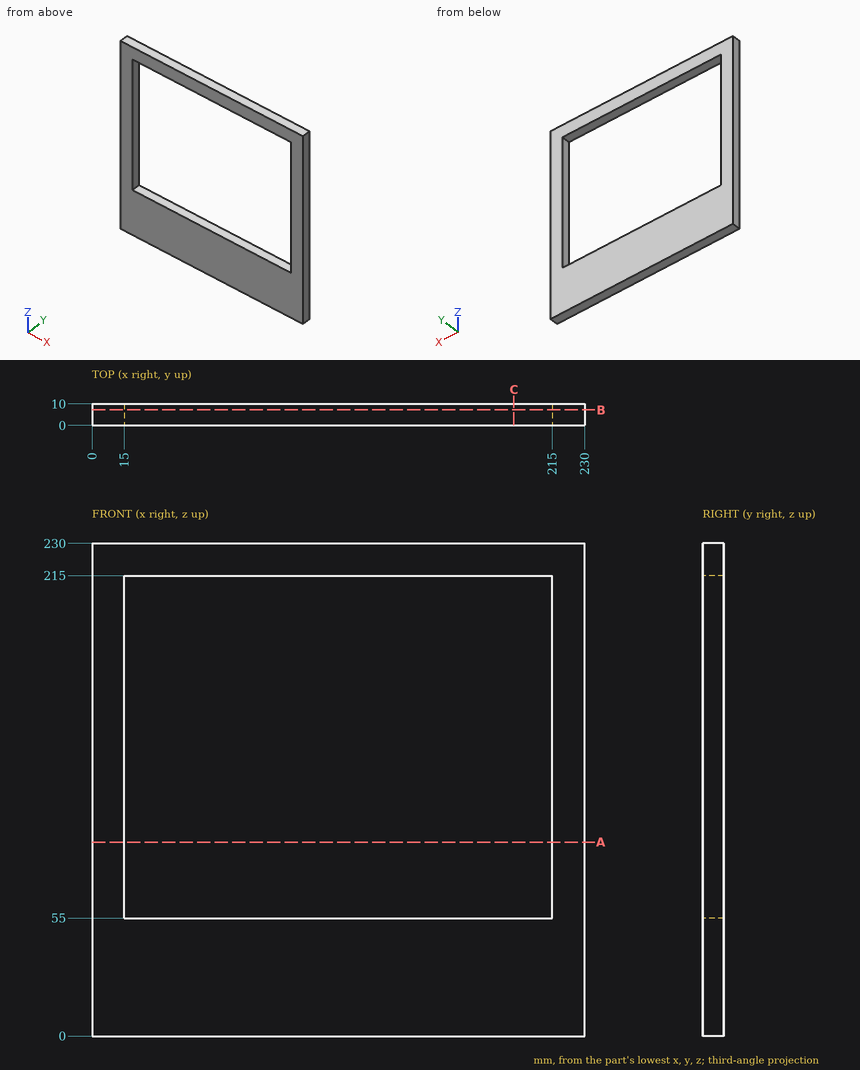
Verification items for this drawing (mm, ordinates from the low corner). Give positions to 0.01 mm unless a question says otherwise; leave off trailing zeros. Write each loop counter-clockwise with the first axis right and the second up, starting at its lowest first coordinate (ties: lowest second). Pieces come first, ordered by that corner, then holes. Notation, with made-up numbers: (83.25, 4.25) -> (140.25, 4.25) arc R26 ccw to (140.25, 21.25) -> close; hole circle Ø10 at (79.25, 6.5). An arc over 180 degrees is marked (long way). Write item = value, one per line.
Item 1: Sectioned sample at A-A on z = 90.5. Record the boundary of the cut face in (x, y), and give its area (3 significant figures).
Output:
outline = (0, 0) -> (15, 0) -> (15, 10) -> (0, 10) -> close; (215, 0) -> (230, 0) -> (230, 10) -> (215, 10) -> close
area = 300 mm^2
Item 2: Sectioned sample at B-B on y = 7.25. Record the boundary of the cut face in (x, z).
Output:
outline = (0, 0) -> (230, 0) -> (230, 230) -> (0, 230) -> close; hole (15, 55) -> (215, 55) -> (215, 215) -> (15, 215) -> close
Item 3: Sectioned sample at C-C on x = 197. Record the boundary of the cut face in (y, z), and give its area (3 significant figures).
Output:
outline = (0, 0) -> (10, 0) -> (10, 55) -> (0, 55) -> close; (0, 215) -> (10, 215) -> (10, 230) -> (0, 230) -> close
area = 700 mm^2
Item 4: Scan lines: probe 1 along X at (y, z) = (4.5, 155.5); probe 2 along Z at (x, y) = (185.5, 8). Record each from-to range of solid material in increasing order. Write a range as from..to.
Output:
probe_1 = 0..15, 215..230
probe_2 = 0..55, 215..230
